Can you work these out from the model? Positions are in its coordinate system, mm. A direction names the side the tool comes from. Round coordinates to 2 decimals unless told otherwise and drop trailing zeros. Order: outer loops, then holes, each group sorted by start corner. A loop starts at its lowest first (then second) coordinate and runs counter-clockwise, first axis right, second up.
Q1. If we section it at D-D (x = -9): Please give me the cut outline in (y, z).
Q2. We'd pull the mould along Z, two halves only. Please class faces 4 (the face through (7.535, 0.67, 1.617)), 5 (the face through (-0.54, -0.07, -2.44)), 6 (the face through (-10, -2, 1)): pulls with the +Z half, pulls with the -Z half, needs draft (parallel to the pull), parting line crosses it, or undercut.
Q3. Will these pins go through, and if not, where does the flat tip stop? P1, Ø2, axis at y = 0.5, z = -1, coming from the -X side; P2, Ø1, axis at y = 3.5, z = 1.5, coming from the +X side; P3, Ø1.5, axis at x = -5.5, y = -2.5, coming from the +Z side; P4, Ø1.5, axis at y = -1, z = 1, coming from the -X side.
Q4. If we section it at A-A (x = 0): Please give me the cut outline in (y, z), plus the area to 3 significant figures.
Q5. If we section it at C-C (z = 1): Please give me the cut outline in (x, y).
Q6. For faces 1 (the face through (-10.3, 2.44, -0.54)), 2 (the face through (10.3, 2.44, -0.54)), 3 (the face through (-7.535, 0.67, 1.617)), which set-ups out of +Z, -Z, +X, -X, +Y, -Y let a thin tool reach every point of the face, with its end or its side?
Q7. If I drill on line 1 (Z direction, x = 0, y = 2.25); line 2 (X direction, y = 2.75, z = 1); line 3 (X direction, y = -0.25, z = -0.25), over which ranges is the centre line in solid material (lowest first)?
Q8. If we section it at B-B (y = 3): Please give me the cut outline in (x, z), plus the area to 3 significant figures.
from build123d import *

# Parameters (mm, degrees)
F1_DEPTH = 5
F0_W     = 5
F0_H     = 1.75
F5_R     = 2.5
F6_DEPTH = 25


# Not quite as in the source:
# - a pattern or mirror of a feature is missing from the dataset's text; its kind, count and spacing are read off the source's solid
# - a feature names something its author has since deleted; it is built from what else it names


with BuildPart() as f1:
    # F0 (on Front) → F1 (new body, symmetric)
    with BuildSketch(Plane.XZ):
        Polygon((5, 1.75), (5, 3.75), (-5, 3.75), (-5, -3.75), (5, -3.75), (5, 0), align=None)
    extrude(amount=F1_DEPTH, both=True)

    # F0 (on Front) → F2 (revolve)
    with BuildSketch(Plane.XZ):
        with Locations((7.5, 0.875)):
            Rectangle(F0_W, F0_H)
    f2 = revolve(axis=Axis((7.5, 0, 0), (1, 0, 0)))

    # F2_copies: F2 across plane
    add(f2.mirror(Plane(origin=(0, 0, 0), x_dir=(0, 0, -1), z_dir=(-1, 0, 0))))

    # F0 (on Front) → F3 (revolve)
    with BuildSketch(Plane.XZ):
        Polygon((10, 2.5), (10, 1.75), (10, 0), (10.6, 0), (10.6, 2.5), align=None)
    f3 = revolve(axis=Axis((12.1656447835, 0, 0), (1, 0, 0)))

    # F3_copies: F3 across plane
    add(f3.mirror(Plane(origin=(0, 0, 0), x_dir=(0, 0, -1), z_dir=(-1, 0, 0))))

    # F0 (on Front) → F4 (revolve)
    with BuildSketch(Plane.XZ):
        with BuildLine():
            Line((10.6, 2.5), (10.6, 0))
            Line((10.6, 0), (11.9, 0))
            ThreePointArc((11.9, 0), (11.5555774622, 1.4089002804), (10.6, 2.5))
        make_face()
    f4 = revolve(axis=Axis((12.1656447835, 0, 0), (1, 0, 0)))

    # F4_copies: F4 across plane
    add(f4.mirror(Plane(origin=(0, 0, 0), x_dir=(0, 0, -1), z_dir=(-1, 0, 0))))

    # F5 (on face) → F6 (cut)
    with BuildSketch(Plane.XZ.offset(5)):
        Circle(F5_R)
    extrude(amount=-F6_DEPTH, mode=Mode.SUBTRACT)


solid = f1.part
Solution:
1. outline: circle Ø3.5 at (0, 0)
2. face 4: parting line crosses it
2. face 5: undercut
2. face 6: needs draft
3. P1: stops at x = -11.9
3. P2: stops at x = 5
3. P3: stops at z = 3.75
3. P4: stops at x = -11.83
4. outline: (-5, -3.75) - (5, -3.75) - (5, -2.5) - (-5, -2.5) - close; (-5, 2.5) - (5, 2.5) - (5, 3.75) - (-5, 3.75) - close
4. area: 25.0 mm2
5. outline: (-10.6, -2.29) - (-10, -2.29) - (-10, -1.44) - (-5, -1.44) - (-5, -5) - (-2.29, -5) - (-2.29, 5) - (-5, 5) - (-5, 1.44) - (-10, 1.44) - (-10, 2.29) - (-10.6, 2.29) arc R2.89 ccw to start; (2.29, -5) - (5, -5) - (5, -1.44) - (10, -1.44) - (10, -2.29) - (10.6, -2.29) arc R2.89 ccw to (10.6, 2.29) - (10, 2.29) - (10, 1.44) - (5, 1.44) - (5, 5) - (2.29, 5) - close
6. face 1: -X
6. face 2: +X
6. face 3: none
7. line 1: z = -3.75 to -2.5, 2.5 to 3.75
7. line 2: x = -5 to -2.29, 2.29 to 5
7. line 3: x = -11.88 to -2.49, 2.49 to 11.88
8. outline: (-5, -3.75) - (5, -3.75) - (5, 3.75) - (-5, 3.75) - close; hole circle Ø5 at (0, 0)
8. area: 55.4 mm2
